Input: part model. Units: mm. Frame: model coordinates. A direction names the side the tool comes from. Coordinates: 2 decimals unless noted, no trailing zeros. Loops run counter-clockwise (first coordinate to the right, second up) from the corner with the lowest first, then second, coordinate; pieces in that order, holes last.
Item 1: Section B-B on y = 175.5. Return loops of the section in (x, z).
Item 2: Reachability of faces 1 (the flat face through (-212.725, 12, 1)), 2 (the cylindrical face through (-213.88, 11.26, -58.79)) from +Z, -Z, +X, -X, +Y, -Y: full face, straight path, thin tool, end or side. Return the list, or none.
Item 3: Ray query, line 1 along X through (y, z) = (17, 26) (3 decimals); line 2 along X through (y, z) = (59.5, 13); line 3 along Y through (x, z) = (0, -11). Return the intervals inside material, ascending.
Item 4: Contact query for flat-ended pins moving along their axis: P1, Ø1.5, axis at x = 83.5, z = -19.5, coming from the -Y side; P2, Ø5, axis at x = -166.5, z = -33.5, coming from the +Y side; P3, Ø1.5, axis at x = -136.5, z = -25, coming from the -Y side. Output: stop coordinate, or through.
Item 5: Pull-direction query (X, two-part tool) for faces 3 (the flat face through (215.9, 12, 1)), 4 (the cylindrical face through (-3.358, 200.784, 0.978)), 5 (the flat face through (199.434, 50.932, 0.978)), 6 (the flat face through (-215.9, 12, 1)); classes: released by +X, released by -X, zero draft, split by the parting line, or undercut.
Item 6: Section D-D on y = 42.5. Return loops of the section in (x, z).
Item 7: Section C-C on x = -124.5. Return loops of the section in (y, z).
```python
from build123d import *

# Parameters (mm, degrees)
BOSS_EXTRUDE1_DEPTH = 69.85
FILLET1_R           = 38.1
FILLET2_R           = 38.1
FILLET3_R           = 38.1
FILLET4_R           = 38.1
FILLET5_R           = 5.08
FILLET6_R           = 5.08


with BuildPart() as part:
    # Sketch2 → Boss-Extrude1 (new, symmetric)
    with BuildSketch(Plane.XY):
        with BuildLine():
            Line((-212.725, 0), (-215.9, 0))
            Line((-215.9, 0), (-215.9, 25.4))
            Line((-215.9, 25.4), (-189.455193832, 76.2))
            ThreePointArc((-189.455193832, 76.2), (0, 200.810907661), (189.455193832, 76.2))
            Line((189.455193832, 76.2), (215.9, 25.4))
            Line((215.9, 25.4), (215.9, 0))
            Line((215.9, 0), (212.725, 0))
            Line((212.725, 0), (212.725, 25.4))
            Line((212.725, 25.4), (186.280193832, 76.2))
            ThreePointArc((186.280193832, 76.2), (0, 197.635907661), (-186.280193832, 76.2))
            Line((-186.280193832, 76.2), (-212.725, 25.4))
            Line((-212.725, 25.4), (-212.725, 0))
        make_face()
    extrude(amount=BOSS_EXTRUDE1_DEPTH, both=True)

    # Fillet1
    # the kernel refuses this fillet: 38.1 mm, written as the material it takes off along each edge
    with BuildSketch(Plane(origin=(311.15, 0, -69.85), x_dir=(0, 1, 0), z_dir=(-1, 0, 0))) as fillet1_piece_1:
        with BuildLine():
            CenterArc((FILLET1_R, -FILLET1_R), FILLET1_R, 90, 90)
            Line((0, -FILLET1_R), (0, 0))
            Line((0, 0), (FILLET1_R, 0))
        make_face()
    extrude(amount=193.675, mode=Mode.SUBTRACT)

    # Fillet2
    # the kernel refuses this fillet: 38.1 mm, written as the material it takes off along each edge
    with BuildSketch(Plane(origin=(311.15, 0, 69.85), x_dir=(0, 0, -1), z_dir=(-1, 0, 0))) as fillet2_piece_1:
        with BuildLine():
            CenterArc((FILLET2_R, -FILLET2_R), FILLET2_R, 90, 90)
            Line((0, -FILLET2_R), (0, 0))
            Line((0, 0), (FILLET2_R, 0))
        make_face()
    extrude(amount=193.675, mode=Mode.SUBTRACT)

    # Fillet3
    # the kernel refuses this fillet: 38.1 mm, written as the material it takes off along each edge
    with BuildSketch(Plane(origin=(-117.475, 0, 69.85), x_dir=(0, 1, 0), z_dir=(-1, 0, 0))) as fillet3_piece_1:
        with BuildLine():
            CenterArc((FILLET3_R, FILLET3_R), FILLET3_R, 180, 90)
            Line((0, FILLET3_R), (0, 0))
            Line((0, 0), (FILLET3_R, 0))
        make_face()
    extrude(amount=193.675, mode=Mode.SUBTRACT)

    # Fillet4
    # the kernel refuses this fillet: 38.1 mm, written as the material it takes off along each edge
    with BuildSketch(Plane(origin=(-117.475, 0, -69.85), x_dir=(0, 1, 0), z_dir=(-1, 0, 0))) as fillet4_piece_1:
        with BuildLine():
            CenterArc((FILLET4_R, -FILLET4_R), FILLET4_R, 90, 90)
            Line((0, -FILLET4_R), (0, 0))
            Line((0, 0), (FILLET4_R, 0))
        make_face()
    extrude(amount=193.675, mode=Mode.SUBTRACT)

    # Fillet5
    fillet5_edges = [part.edges().sort_by_distance(p)[0] for p in [
        (215.9, 25.4, 0),
        (-215.9, 25.4, 0),
        (-212.725, 25.4, 0),
        (212.725, 25.4, 0),
    ]]
    fillet(fillet5_edges, radius=FILLET5_R)

    # Fillet6
    # the kernel refuses this fillet: 5.08 mm, written as the material it adds along each edge
    with BuildSketch(Plane(origin=(-189.455193832, 76.2, 69.85), x_dir=(0.3964547937843397, 0.9180542448490813, 0), z_dir=(0, 0, -1))) as fillet6_piece_1:
        with BuildLine():
            CenterArc((0.183763375, -5.079999508), FILLET6_R, 90.025204734, 4.118058509)
            Line((-0.183269559, -0.013276028), (0, 0))
            ThreePointArc((0, 0), (0.090764327, -1.9964e-05), (0.181528655, 0))
        make_face()
    extrude(amount=139.7)
    with BuildSketch(Plane(origin=(189.455193832, 76.2, 69.85), x_dir=(0.4617486132350293, -0.887010833178224, 0), z_dir=(0, 0, -1))) as fillet6_piece_2:
        with BuildLine():
            CenterArc((0.183749786, -5.08), FILLET6_R, 90, 4.118058509)
            ThreePointArc((-0.181054232, -0.01311555), (-0.090525673, -0.006577687), (0, 0))
            Line((0, 0), (0.183749786, 0))
        make_face()
    extrude(amount=139.7)
    # the kernel refuses this fillet: 5.08 mm, written as the material it takes off along each edge
    with BuildSketch(Plane(origin=(186.280193832, 76.2, 70.257743197), x_dir=(0.4617486132350699, -0.8870108331782028, 0), z_dir=(0, 0, -1))) as fillet6_2_piece_1:
        with BuildLine():
            CenterArc((0.163097279, -5.08), FILLET6_R, 90, 3.655257242)
            ThreePointArc((-0.160768001, -0.010334204), (-0.080382979, -0.005183004), (0, 0))
            Line((0, 0), (0.163097279, 0))
        make_face()
    extrude(amount=140.515486395, mode=Mode.SUBTRACT)
    with BuildSketch(Plane(origin=(-186.280193832, 76.2, 70.257743197), x_dir=(-0.46174861323509436, -0.8870108331781903, 0), z_dir=(0, 0, -1))) as fillet6_2_piece_2:
        with BuildLine():
            CenterArc((0.163097279, 5.08), FILLET6_R, 266.344742758, 3.655257242)
            ThreePointArc((-0.160768001, 0.010334204), (-0.080382979, 0.005183004), (0, 0))
            Line((0, 0), (0.163097279, 0))
        make_face()
    extrude(amount=140.515486395, mode=Mode.SUBTRACT)


solid = part.part
```
Results found:
1. outline: (-99.02, -69.85) - (-92.32, -69.85) - (-92.32, 69.85) - (-99.02, 69.85) - close; (92.32, -69.85) - (99.02, -69.85) - (99.02, 69.85) - (92.32, 69.85) - close
2. face 1: +Z, -Z, -Y
2. face 2: -Z, +X, -X, -Y
3. line 1: x = -215.9 to -212.725, 212.725 to 215.9
3. line 2: x = -198.15 to -194.97, 194.97 to 198.15
3. line 3: y = 197.64 to 200.81
4. P1: stops at y = 179.39
4. P2: stops at y = 119.68
4. P3: stops at y = 144.42
5. face 3: released by +X
5. face 4: split by the parting line
5. face 5: undercut
5. face 6: released by -X
6. outline: (-207, -69.85) - (-203.82, -69.85) - (-203.82, 69.85) - (-207, 69.85) - close; (203.82, -69.85) - (207, -69.85) - (207, 69.85) - (203.82, 69.85) - close
7. outline: (155.13, -69.85) - (159.02, -69.85) - (159.02, 69.85) - (155.13, 69.85) - close
